Source: CAD feature listing. Evaluate the final solid. Frame: model axes, mm. A direction names the side the tool comes from. Give positions to 0.01 mm unless a question says otherwise; leave off trailing zeros. Order: outer loops, then holes, each group sorted by start corner. A loop starts at its lowest first (then second) coordinate and runs counter-clockwise, first axis right, second up.
1) Section A-A, the plane y = 10.5. Return loops of the section in (x, z), plus the area to 3 significant figures.
2) Section B-B, the plane z = 0. Return loops of the section in (x, y), plus the area to 3 significant figures.
3) Access query for faces 5 (the face through (-13, 3, 7)), 6 (the face through (-0.3, 2.5, 1.545)), 7 (the face through (-23.88, 19.1, 2)), 8 (the face through (0, 1.6, -6)). Directions: +Z, -Z, +X, -X, +Y, -Y. A direction counts if a zero-diameter tool reaches every point of the face in a straight line with its end or side. Return the directions, or none.
4) Material intervals for line 1 (X direction, y = 2.75, z = -8.5); line 2 (X direction, y = 22.5, z = 6.75); line 3 (X direction, y = 21, z = -3), sorted ascending.
5) Draft query along Z for faces 1 (the face through (0, 3.5, 6)), 2 (the face through (23.898, 13.031, -5.645)), 3 (the face through (-23.862, 21.227, -8.935)), 4 (the face through (-23.862, 21.141, 8.966)). Return one class per face: released by +Z, released by -Z, zero draft, split by the parting line, or undercut.
6) Section C-C, the plane y = 17. Return loops of the section in (x, z), plus the area to 3 significant figures.
7) First-contact query: P1, Ø0.5, axis at x = 3, z = 1, coming from the +Y side; P2, Ø3, axis at x = -24, z = 0.5, coming from the +Y side; P3, Ø1, axis at x = -1.5, z = -8.5, coming from the +Y side. Flat tips, straight axial feed; report the tip coordinate or a pass-through.
```python
from build123d import *

# Parameters (mm, degrees)
SKETCH1_W           = 50.26
SKETCH1_H           = 24
BOSS_EXTRUDE1_DEPTH = 2
SKETCH2_W           = 2.5
SKETCH2_H           = 24
BOSS_EXTRUDE2_DEPTH = 22
SKETCH3_R           = 2.1
CUT_EXTRUDE1_DEPTH  = 57.974271386
SKETCH4_R           = 4.7
CUT_EXTRUDE2_DEPTH  = 1.25
CUT_EXTRUDE3_REACH  = 58.974
SKETCH5_R           = 1.25
CUT_EXTRUDE4_REACH  = 58.974
SKETCH7_W           = 45.26
SKETCH7_H           = 1
BOSS_EXTRUDE3_DEPTH = 1
LPATTERN3_COUNT     = 12
LPATTERN3_PITCH     = 2.090909091
BOSS_EXTRUDE4_DEPTH = 2.5
CUT_EXTRUDE6_DEPTH  = 59.424713631
BOSS_EXTRUDE5_START = -1
SKETCH12_W          = 7
SKETCH12_H          = 3.5
BOSS_EXTRUDE5_DEPTH = 3
SKETCH13_R          = 0.925
CUT_EXTRUDE7_DEPTH  = 3.5
CUT_EXTRUDE9_START  = -3.5
SKETCH14_R          = 0.925
CUT_EXTRUDE9_DEPTH  = 3.5


with BuildPart() as part:
    # Sketch1 → Boss-Extrude1 (new body)
    with BuildSketch(Plane(origin=(0, 0, 0), x_dir=(1, 0, 0), z_dir=(0, 1, 0))):
        Rectangle(SKETCH1_W, SKETCH1_H)
    extrude(amount=BOSS_EXTRUDE1_DEPTH)

    # Sketch2 → Boss-Extrude2 (add)
    with BuildSketch(Plane(origin=(0, 2, 0), x_dir=(1, 0, 0), z_dir=(0, 1, 0))):
        with Locations((-23.88, 0)):
            Rectangle(SKETCH2_W, SKETCH2_H)
        with Locations((23.88, 0)):
            Rectangle(SKETCH2_W, SKETCH2_H)
    extrude(amount=BOSS_EXTRUDE2_DEPTH)

    # Sketch3 → Cut-Extrude1 (cut, through all)
    with BuildSketch(Plane(origin=(25.13, 0, 0), x_dir=(0, 0, -1), z_dir=(1, 0, 0))):
        with Locations((0, 18)):
            Circle(SKETCH3_R)
    extrude(amount=-CUT_EXTRUDE1_DEPTH, mode=Mode.SUBTRACT)

    # Sketch4 → Cut-Extrude2 (cut)
    with BuildSketch(Plane.ZY.offset(-22.63)):
        with Locations((0, 18)):
            Circle(SKETCH4_R)
    cut_extrude2 = extrude(amount=-CUT_EXTRUDE2_DEPTH, mode=Mode.SUBTRACT)

    # Mirror1: Cut-Extrude2 across plane
    add(cut_extrude2.mirror(Plane.ZY), mode=Mode.SUBTRACT)

    # Sketch5 → Cut-Extrude3 (cut, up to next)
    with BuildSketch(Plane(origin=(25.13, 0, 0), x_dir=(0, 0, -1), z_dir=(1, 0, 0)), mode=Mode.PRIVATE) as cut_extrude3_sk1:
        with Locations((4.49015, 13.50985)):
            Circle(SKETCH5_R)
    cut_extrude3_tool1 = extrude(cut_extrude3_sk1.sketch, amount=-CUT_EXTRUDE3_REACH, mode=Mode.PRIVATE) & part.part
    # Sketch5 → Cut-Extrude3 (cut, up to next)
    with BuildSketch(Plane(origin=(25.13, 0, 0), x_dir=(0, 0, -1), z_dir=(1, 0, 0)), mode=Mode.PRIVATE) as cut_extrude3_sk2:
        with Locations((-4.49015, 13.50985)):
            Circle(SKETCH5_R)
    cut_extrude3_tool2 = extrude(cut_extrude3_sk2.sketch, amount=-CUT_EXTRUDE3_REACH, mode=Mode.PRIVATE) & part.part
    # Sketch5 → Cut-Extrude3 (cut, up to next)
    with BuildSketch(Plane(origin=(25.13, 0, 0), x_dir=(0, 0, -1), z_dir=(1, 0, 0)), mode=Mode.PRIVATE) as cut_extrude3_sk3:
        with Locations((-4.49015, 22.49015)):
            Circle(SKETCH5_R)
    cut_extrude3_tool3 = extrude(cut_extrude3_sk3.sketch, amount=-CUT_EXTRUDE3_REACH, mode=Mode.PRIVATE) & part.part
    # Sketch5 → Cut-Extrude3 (cut, up to next)
    with BuildSketch(Plane(origin=(25.13, 0, 0), x_dir=(0, 0, -1), z_dir=(1, 0, 0)), mode=Mode.PRIVATE) as cut_extrude3_sk4:
        with Locations((4.49015, 22.49015)):
            Circle(SKETCH5_R)
    cut_extrude3_tool4 = extrude(cut_extrude3_sk4.sketch, amount=-CUT_EXTRUDE3_REACH, mode=Mode.PRIVATE) & part.part
    add(cut_extrude3_tool1.solids().sort_by_distance((25.13, 13.50985, -4.49015))[0], mode=Mode.SUBTRACT)
    add(cut_extrude3_tool2.solids().sort_by_distance((25.13, 13.50985, 4.49015))[0], mode=Mode.SUBTRACT)
    add(cut_extrude3_tool3.solids().sort_by_distance((25.13, 22.49015, 4.49015))[0], mode=Mode.SUBTRACT)
    add(cut_extrude3_tool4.solids().sort_by_distance((25.13, 22.49015, -4.49015))[0], mode=Mode.SUBTRACT)

    # Sketch6 → Cut-Extrude4 (cut, up to next)
    with BuildSketch(Plane(origin=(25.13, 0, 0), x_dir=(0, 0, -1), z_dir=(1, 0, 0)), mode=Mode.PRIVATE) as cut_extrude4_sk1:
        with BuildLine():
            Line((-2.1, 18), (-2.1, 24))
            Line((-2.1, 24), (2.1, 24))
            Line((2.1, 24), (2.1, 18))
            ThreePointArc((2.1, 18), (0, 15.9), (-2.1, 18))
        make_face()
    cut_extrude4_tool1 = extrude(cut_extrude4_sk1.sketch, amount=-CUT_EXTRUDE4_REACH, mode=Mode.PRIVATE) & part.part
    add(cut_extrude4_tool1.solids().sort_by_distance((25.13, 20.160972, 0))[0], mode=Mode.SUBTRACT)

    # Sketch7 → Boss-Extrude3 (add)
    with BuildSketch(Plane(origin=(0, 2, 0), x_dir=(1, 0, 0), z_dir=(0, 1, 0))):
        with Locations((0, -11.5)):
            Rectangle(SKETCH7_W, SKETCH7_H)
    boss_extrude3 = extrude(amount=BOSS_EXTRUDE3_DEPTH)

    # LPattern3: Boss-Extrude3 ×12
    with Locations(*[(0, 0, -i * LPATTERN3_PITCH) for i in range(1, LPATTERN3_COUNT)]):
        add(boss_extrude3)

    # Sketch9 → Boss-Extrude4 (add)
    with BuildSketch(Plane(origin=(25.13, 0, 0), x_dir=(0, 0, -1), z_dir=(1, 0, 0))):
        with BuildLine():
            Line((2.1, 24), (7.365459931, 24))
            ThreePointArc((7.365459931, 24), (5.006372874, 26.073799022), (2.1, 27.264987858))
            Line((2.1, 27.264987858), (2.1, 24))
        make_face()
        with BuildLine():
            Line((-7.365459931, 24), (-2.1, 24))
            Line((-2.1, 24), (-2.1, 27.264987858))
            ThreePointArc((-2.1, 27.264987858), (-5.006372874, 26.073799022), (-7.365459931, 24))
        make_face()
    extrude(amount=-BOSS_EXTRUDE4_DEPTH)

    # Sketch10 → Cut-Extrude6 (cut, through all)
    with BuildSketch(Plane(origin=(25.13, 0, 0), x_dir=(0, 0, -1), z_dir=(1, 0, 0))):
        with BuildLine():
            Line((-9.5, 0), (-9.5, 18))
            ThreePointArc((-9.5, 18), (-8.950471198, 21.184189901), (-7.365459931, 24))
            Line((-7.365459931, 24), (-9.5, 24))
            Line((-9.5, 24), (-12, 24))
            Line((-12, 24), (-12, 0))
            Line((-12, 0), (-9.5, 0))
        make_face()
        with BuildLine():
            Line((9.5, 24), (7.365459931, 24))
            ThreePointArc((7.365459931, 24), (8.950471198, 21.184189901), (9.5, 18))
            Line((9.5, 18), (9.5, 0))
            Line((9.5, 0), (12, 0))
            Line((12, 0), (12, 24))
            Line((12, 24), (9.5, 24))
        make_face()
    extrude(amount=-CUT_EXTRUDE6_DEPTH, mode=Mode.SUBTRACT)

    # Sketch12 → Boss-Extrude5 (add)
    with BuildSketch(Plane(origin=(0, 3, 0), x_dir=(1, 0, 0), z_dir=(0, 1, 0)).offset(BOSS_EXTRUDE5_START)):
        with Locations((0, -7.75)):
            Rectangle(SKETCH12_W, SKETCH12_H)
    boss_extrude5 = extrude(amount=BOSS_EXTRUDE5_DEPTH)

    # Mirror2: Boss-Extrude5 across plane
    add(boss_extrude5.mirror(Plane.XY))

    # Sketch13 → Cut-Extrude7 (cut)
    with BuildSketch(Plane(origin=(0, 0, -9.5), x_dir=(-1, 0, 0), z_dir=(0, 0, -1))):
        with Locations(Location((0, 2, 0), (0, 0, 90))):
            Circle(SKETCH13_R)
    extrude(amount=-CUT_EXTRUDE7_DEPTH, mode=Mode.SUBTRACT)

    # Sketch14 → Cut-Extrude9 (cut)
    with BuildSketch(Plane.XY.offset(9.5).offset(CUT_EXTRUDE9_START)):
        with Locations(Location((0, 2, 0), (0, 0, 90))):
            Circle(SKETCH14_R)
    extrude(amount=CUT_EXTRUDE9_DEPTH, mode=Mode.SUBTRACT)


solid = part.part
```
From the geometry:
1. outline: (-25.13, -9.5) - (-22.63, -9.5) - (-22.63, 9.5) - (-25.13, 9.5) - close; (22.63, -9.5) - (25.13, -9.5) - (25.13, 9.5) - (22.63, 9.5) - close
1. area: 95.0 mm2
2. outline: (-25.13, 0) - (25.13, 0) - (25.13, 15.9) - (23.88, 15.9) - (23.88, 13.3) - (22.63, 13.3) - (22.63, 2) - (-22.63, 2) - (-22.63, 13.3) - (-23.88, 13.3) - (-23.88, 15.9) - (-25.13, 15.9) - close; (-25.13, 20.1) - (-23.88, 20.1) - (-23.88, 22.7) - (-22.63, 22.7) - (-22.63, 24) - (-25.13, 24) - close
2. area: 170 mm2
3. face 5: +Z, -Z, +Y
3. face 6: +Y
3. face 7: none
3. face 8: -Z
4. line 1: x = -25.13 to -22.63, -3.5 to -0.54, 0.54 to 3.5, 22.63 to 25.13
4. line 2: x = -25.13 to -22.63, 22.63 to 25.13
4. line 3: x = -25.13 to -23.88, 23.88 to 25.13
5. face 1: undercut
5. face 2: undercut
5. face 3: released by -Z
5. face 4: released by +Z
6. outline: (-25.13, -9.5) - (-22.63, -9.5) - (-22.63, -4.59) - (-23.88, -4.59) - (-23.88, -1.85) - (-25.13, -1.85) - close; (-25.13, 1.85) - (-23.88, 1.85) - (-23.88, 4.59) - (-22.63, 4.59) - (-22.63, 9.5) - (-25.13, 9.5) - close; (22.63, -9.5) - (25.13, -9.5) - (25.13, -1.85) - (23.88, -1.85) - (23.88, -4.59) - (22.63, -4.59) - close; (22.63, 4.59) - (23.88, 4.59) - (23.88, 1.85) - (25.13, 1.85) - (25.13, 9.5) - (22.63, 9.5) - close
6. area: 62.8 mm2
7. P1: stops at y = 3
7. P2: stops at y = 24
7. P3: stops at y = 5
